Source: CAD feature listing. Evaluate the final solid. Frame: model axes, mm. A direction names the side the tool comes from. Coordinates: 2 decimals unless noted, no trailing zeros. Order: outer loops, then holes, each group sorted by start corner. A loop starts at its lowest first (then second) coordinate and runs counter-clockwise, first axis right, second up. Notation, with made-up numbers: (-3.75, 0) -> (31.25, 0) arc R23 ccw to (31.25, 8) -> close; hole circle Ø1 at (-5, -28). An arc over 180 degrees is marked (long way). Put each result on its own line as item: value.
from build123d import *

# Parameters (mm, degrees)
SKETCH1_W           = 62.5
SKETCH1_H           = 45
BOSS_EXTRUDE1_DEPTH = 20
SKETCH2_W           = 37.5
SKETCH2_H           = 45
CUT_EXTRUDE1_DEPTH  = 5
SKETCH3_R           = 11.5
CUT_EXTRUDE2_DEPTH  = 2
SKETCH4_R           = 1.5
CUT_EXTRUDE3_DEPTH  = 15
CIRPATTERN1_COUNT   = 4
SKETCH5_R           = 2.75
CUT_EXTRUDE4_DEPTH  = 58.66769
CUT_EXTRUDE7_START  = -6.5
CUT_EXTRUDE7_DEPTH  = 3
CUT_EXTRUDE8_DEPTH  = 6.5
CUT_EXTRUDE9_DEPTH  = 5.5
SKETCH11_R          = 1.375
CUT_EXTRUDE10_DEPTH = 80.569152
FILLET1_R           = 2
SKETCH12_R          = 3.625
CUT_EXTRUDE12_DEPTH = 3
BOSS_EXTRUDE2_START = 20
BOSS_EXTRUDE2_DEPTH = 20
SKETCH14_R          = 4
CUT_EXTRUDE18_DEPTH = 2
SKETCH15_W          = 62.5
SKETCH15_H          = 45
CUT_EXTRUDE19_DEPTH = 7
SKETCH16_R          = 3.25
CUT_EXTRUDE20_DEPTH = 64.957506
SKETCH17_R          = 1.375
CUT_EXTRUDE21_DEPTH = 79.008013


with BuildPart() as part:
    # Sketch1 → Boss-Extrude1 (new body)
    with BuildSketch(Plane.XY):
        with Locations((0, 22.5)):
            Rectangle(SKETCH1_W, SKETCH1_H)
    extrude(amount=BOSS_EXTRUDE1_DEPTH)

    # Sketch2 → Cut-Extrude1 (cut)
    with BuildSketch(Plane.XY.offset(20)):
        with Locations((0, 22.5)):
            Rectangle(SKETCH2_W, SKETCH2_H)
    extrude(amount=-CUT_EXTRUDE1_DEPTH, mode=Mode.SUBTRACT)

    # Sketch3 → Cut-Extrude2 (cut)
    with BuildSketch(Plane(origin=(0, 0, 0), x_dir=(-1, 0, 0), z_dir=(0, 0, -1))):
        with Locations((0, 27.5)):
            Circle(SKETCH3_R)
    extrude(amount=-CUT_EXTRUDE2_DEPTH, mode=Mode.SUBTRACT)

    # Sketch4 → Cut-Extrude3 (cut)
    with BuildSketch(Plane(origin=(0, 0, 0), x_dir=(-1, 0, 0), z_dir=(0, 0, -1))):
        with Locations((11.5, 39)):
            Circle(SKETCH4_R)
    cut_extrude3 = extrude(amount=-CUT_EXTRUDE3_DEPTH, mode=Mode.SUBTRACT)

    # CirPattern1: Cut-Extrude3 ×4 about axis
    cirpattern1_axis = Axis((0, 27.5, 0), (0, 0, 1))
    for i in range(1, CIRPATTERN1_COUNT):
        add(cut_extrude3.rotate(cirpattern1_axis, i * 360 / CIRPATTERN1_COUNT), mode=Mode.SUBTRACT)

    # Sketch5 → Cut-Extrude4 (cut, through all)
    with BuildSketch(Plane(origin=(0, 0, 2), x_dir=(-1, 0, 0), z_dir=(0, 0, -1))):
        with Locations((0, 27.5)):
            Circle(SKETCH5_R)
    extrude(amount=-CUT_EXTRUDE4_DEPTH, mode=Mode.SUBTRACT)

    # Sketch8 → Cut-Extrude7 (cut)
    with BuildSketch(Plane(origin=(0, 0, 0), x_dir=(-1, 0, 0), z_dir=(0, 0, -1)).offset(CUT_EXTRUDE7_START)):
        with BuildLine():
            Line((7.125, 0), (-7.125, 0))
            Line((-7.125, 0), (-7.125, 11.75))
            ThreePointArc((-7.125, 11.75), (-6.539214, 13.164214), (-5.125, 13.75))
            Line((-5.125, 13.75), (5.125, 13.75))
            ThreePointArc((5.125, 13.75), (6.539214, 13.164214), (7.125, 11.75))
            Line((7.125, 11.75), (7.125, 0))
        make_face()
    extrude(amount=-CUT_EXTRUDE7_DEPTH, mode=Mode.SUBTRACT)

    # Sketch9 → Cut-Extrude8 (cut)
    with BuildSketch(Plane(origin=(0, 0, 0), x_dir=(-1, 0, 0), z_dir=(0, 0, -1))):
        with BuildLine():
            Line((4.75, 7.5), (4.75, 0))
            Line((4.75, 0), (-4.75, 0))
            Line((-4.75, 0), (-4.75, 7.5))
            ThreePointArc((-4.75, 7.5), (0, 12.25), (4.75, 7.5))
        make_face()
    extrude(amount=-CUT_EXTRUDE8_DEPTH, mode=Mode.SUBTRACT)

    # Sketch10 → Cut-Extrude9 (cut)
    with BuildSketch(Plane.XY.offset(15)):
        with BuildLine():
            Line((2.575, 7.5), (2.575, 0))
            Line((2.575, 0), (-2.575, 0))
            Line((-2.575, 0), (-2.575, 7.5))
            ThreePointArc((-2.575, 7.5), (0, 10.075), (2.575, 7.5))
        make_face()
    extrude(amount=-CUT_EXTRUDE9_DEPTH, mode=Mode.SUBTRACT)

    # Sketch11 → Cut-Extrude10 (cut, through all)
    with BuildSketch(Plane(origin=(31.25, 0, 0), x_dir=(0, 0, -1), z_dir=(1, 0, 0))):
        with Locations(Location((-17.5, 2.5, 0), (0, 0, 90))):
            Circle(SKETCH11_R)
    extrude(amount=-CUT_EXTRUDE10_DEPTH, mode=Mode.SUBTRACT)

    # Fillet1
    # the kernel refuses this fillet: 2 mm, written as the material it takes off along each edge
    with BuildSketch(Plane(origin=(31.25, 0, -5), x_dir=(0, 1, 0), z_dir=(0, 0, 1)), Plane(origin=(-31.25, 0, -5), x_dir=(1, 0, 0), z_dir=(0, 0, 1))) as fillet1_piece_1:
        with BuildLine():
            CenterArc((FILLET1_R, FILLET1_R), FILLET1_R, 180, 90)
            Line((0, FILLET1_R), (0, 0))
            Line((0, 0), (FILLET1_R, 0))
        make_face()
    extrude(amount=30, mode=Mode.SUBTRACT)

    # Sketch12 → Cut-Extrude12 (cut)
    with BuildSketch(Plane(origin=(31.25, 0, 0), x_dir=(0, 0, -1), z_dir=(1, 0, 0))):
        with Locations((-17.5, 2.5)):
            Circle(SKETCH12_R)
    cut_extrude12 = extrude(amount=-CUT_EXTRUDE12_DEPTH, mode=Mode.SUBTRACT)

    # Mirror3: Cut-Extrude12 across plane
    add(cut_extrude12.mirror(Plane(origin=(0, 0, 0), x_dir=(0, 0, 1), z_dir=(1, 0, 0))), mode=Mode.SUBTRACT)

    # Sketch13 → Boss-Extrude2 (add)
    with BuildSketch(Plane(origin=(0, 0, 0), x_dir=(-1, 0, 0), z_dir=(0, 0, -1)).offset(BOSS_EXTRUDE2_START)):
        with BuildLine():
            Line((17.93986, 0), (29.25, 0))
            ThreePointArc((29.25, 0), (30.664214, 0.585786), (31.25, 2))
            Line((31.25, 2), (31.25, 45))
            Line((31.25, 45), (17.93986, 45))
            Line((17.93986, 45), (17.93986, 0))
        make_face()
    boss_extrude2 = extrude(amount=-BOSS_EXTRUDE2_DEPTH)

    # Sketch14 → Cut-Extrude18 (cut)
    with BuildSketch(Plane.ZY.offset(31.25)):
        with BuildLine():
            ThreePointArc((-20, 3.891941), (-20.187004, 3.207107), (-20.25, 2.5))
            ThreePointArc((-20.25, 2.5), (-19.588022, 0.296002), (-17.821195, -1.178498))
            ThreePointArc((-17.821195, -1.178498), (-14.259364, -0.969491), (-12.281373, 2))
            Line((-12.281373, 2), (-20, 2))
            Line((-20, 2), (-20, 3.891941))
        make_face()
        with BuildLine():
            ThreePointArc((-12.25, 2.5), (-15.542893, 6.437004), (-20, 3.891941))
            Line((-20, 3.891941), (-20, 2))
            Line((-20, 2), (-12.281373, 2))
            ThreePointArc((-12.281373, 2), (-12.257851, 2.249508), (-12.25, 2.5))
        make_face()
        with BuildLine():
            ThreePointArc((-17.821195, -1.178498), (-19.588022, 0.296002), (-20.25, 2.5))
            Line((-20.25, 2.5), (-20.25, -1.178498))
            Line((-20.25, -1.178498), (-17.821195, -1.178498))
        make_face()
        with Locations((-6.25, 2.5)):
            Circle(SKETCH14_R)
    cut_extrude18 = extrude(amount=-CUT_EXTRUDE18_DEPTH, mode=Mode.SUBTRACT)

    # Sketch15 → Cut-Extrude19 (cut)
    with BuildSketch(Plane.XY.offset(20)):
        with Locations((0, 22.5)):
            Rectangle(SKETCH15_W, SKETCH15_H)
    extrude(amount=-CUT_EXTRUDE19_DEPTH, mode=Mode.SUBTRACT)

    # Sketch16 → Cut-Extrude20 (cut, through all)
    with BuildSketch(Plane.XY.offset(13)):
        with BuildLine():
            Line((-24.625, 0), (-24.625, 4.271707))
            ThreePointArc((-24.625, 4.271707), (-25, 4.25), (-25.375, 4.271707))
            Line((-25.375, 4.271707), (-25.375, 0))
            Line((-25.375, 0), (-24.625, 0))
        make_face()
        with Locations((-25, 7.5)):
            Circle(SKETCH16_R)
    cut_extrude20 = extrude(amount=-CUT_EXTRUDE20_DEPTH, mode=Mode.SUBTRACT)

    # Mirror4: Boss-Extrude2, Cut-Extrude18, Cut-Extrude20 across plane
    add(boss_extrude2.mirror(Plane(origin=(0, 0, 0), x_dir=(0, 0, 1), z_dir=(1, 0, 0))))
    add(cut_extrude18.mirror(Plane(origin=(0, 0, 0), x_dir=(0, 0, 1), z_dir=(1, 0, 0))), mode=Mode.SUBTRACT)
    add(cut_extrude20.mirror(Plane(origin=(0, 0, 0), x_dir=(0, 0, 1), z_dir=(1, 0, 0))), mode=Mode.SUBTRACT)

    # Sketch17 → Cut-Extrude21 (cut, through all)
    with BuildSketch(Plane.ZY.offset(29.25)):
        with Locations(Location((-6.25, 2.5, 0), (0, 0, 180))):
            Circle(SKETCH17_R)
        with Locations(Location((-16.25, 2.5, 0), (0, 0, 180))):
            Circle(SKETCH17_R)
    extrude(amount=-CUT_EXTRUDE21_DEPTH, mode=Mode.SUBTRACT)


solid = part.part
1. Pull-direction query (X, two-part tool) for faces 5 (the cylindrical face through (21.236, 2.44, -14.876)), 6 (the cylindrical face through (0.358, 30.227, 7.423)), 7 (the flat face through (-4.75, 4, 3)), 8 (the flat face through (31.25, 23, -4)); classes: pulls with the +X half, pulls with the -X half, needs draft (parallel to the pull), parting line crosses it, or undercut.
Numbers:
face 5: needs draft
face 6: undercut
face 7: undercut
face 8: pulls with the +X half
2. Cut plane A-A on x = 0. Output: boundary loops of the cut face in (y, z) (3 decimals), plus the area to 3 significant figures.
Numbers:
outline: (10.075, 9.5) -> (13.75, 9.5) -> (13.75, 6.5) -> (12.25, 6.5) -> (12.25, 0) -> (16, 0) -> (16, 2) -> (24.75, 2) -> (24.75, 13) -> (10.075, 13) -> close; (30.25, 2) -> (39, 2) -> (39, 0) -> (45, 0) -> (45, 13) -> (30.25, 13) -> close
area: 322 mm2
3. Cut plane C-C on z = 4. Output: boundary loops of the cut face in (x, y) (3 decimals), plus the area to 3 significant figures.
Numbers:
outline: (-31.25, 2) arc R2 ccw to (-29.25, 0) -> (-25.375, 0) -> (-25.375, 4.272) arc R3.25 cw (long way) to (-24.625, 4.272) -> (-24.625, 0) -> (-4.75, 0) -> (-4.75, 7.5) arc R4.75 cw to (4.75, 7.5) -> (4.75, 0) -> (24.625, 0) -> (24.625, 4.272) arc R3.25 cw (long way) to (25.375, 4.272) -> (25.375, 0) -> (29.25, 0) arc R2 ccw to (31.25, 2) -> (31.25, 45) -> (-31.25, 45) -> close; hole circle Ø3 at (-11.5, 16); hole circle Ø3 at (-11.5, 39); hole circle Ø5.5 at (0, 27.5); hole circle Ø3 at (11.5, 16); hole circle Ø3 at (11.5, 39)
area: 2,580 mm2
4. Cut plane D-D on z = -16.25. Count the separate pieces of the cut face and the enclosed holes in it, plus the area to 3 significant figures.
Numbers:
separate pieces: 6
enclosed holes: 0
area: 1,040 mm2
5. First-contact query: pin 1 (2.5 mm diameter, centred on y = 2.5, z = -16.25, fed in from -X); pin 2 (3.5 mm diameter, centred on y = 2.5, z = -7.5, fed in from +X); pin 3 (6 mm diameter, centred on x = 2, y = 20.5, fed in from -Z); pin 4 (5 mm diameter, centred on x = 14, y = 37, fed in from -Z). Flat tips, straight axial feed; report the tip coordinate or a pass-through.
Numbers:
pin 1: passes through
pin 2: stops at x = 29.25
pin 3: stops at z = 2
pin 4: stops at z = 0
6. Set-up query: faces 1 (the cylindrical face through (-30.264, 6.498, -6.124)), 2 (the flat face through (-2, 25, 2)), 3 (the flat face through (0, 13.75, 8)), 4 (the cylindrical face through (-30.042, 1.155, -12.483)). Return all of +Z, -Z, +X, -X, +Y, -Y with unobstructed straight access to the full face (end or side cutting, diameter ignored); none if empty.
Numbers:
face 1: -X
face 2: -Z
face 3: -Y
face 4: -Z, -X
7. Ray query, line 1 along Z through (x, y) = (21, 2.5) (3 decimals); line 2 along X through (y, z) = (12, -11); line 3 along Y through (x, z) = (-28.5, -6.25) (3 decimals). Return the intervals inside material, ascending.
Numbers:
line 1: z = -20 to -17.625, -14.875 to -7.625, -4.875 to 13
line 2: x = -31.25 to -17.94, 17.94 to 31.25
line 3: y = 0 to 1.125, 3.875 to 45
8. Cut plane B-B on y = 27.5. Output: boundary loops of the cut face in (x, z), plus the area to 3 significant figures.
Numbers:
outline: (-31.25, -20) -> (-17.94, -20) -> (-17.94, 0) -> (-11.5, 0) -> (-11.5, 2) -> (-2.75, 2) -> (-2.75, 13) -> (-31.25, 13) -> close; (2.75, 2) -> (11.5, 2) -> (11.5, 0) -> (17.94, 0) -> (17.94, -20) -> (31.25, -20) -> (31.25, 13) -> (2.75, 13) -> close
area: 1,240 mm2
